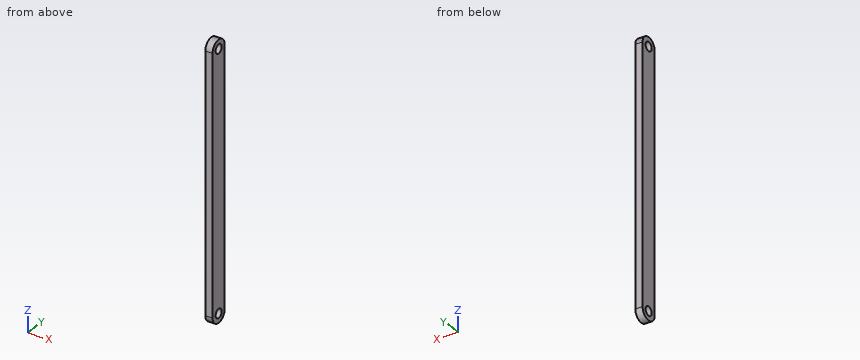
Autodesk Inventor part; units mm, degrees
ref_plane "YZ Plane" through (0, 0, 0) normal (1, 0, 0) x (0, 1, 0)
ref_plane "XZ Plane" through (0, 0, 0) normal (0, 1, 0) x (-1, 0, 0)
ref_plane "XY Plane" through (0, 0, 0) normal (0, 0, 1) x (1, 0, 0)
sketch "Sketch1" plane through (0, 0, 0) normal (1, 0, 0) x (0, 1, 0)
  line L0 (0, 0) -> (0, -70)
  arc A0 (2.5, 0) -> (-2.5, 0) centre (0, 0) ccw
  arc A1 (-2.5, -70) -> (2.5, -70) centre (0, -70) ccw
  line L1 (2.5, 0) -> (2.5, -70)
  line L2 (-2.5, 0) -> (-2.5, -70)
  circle A2 centre (0, 0) radius 1.25
  circle A3 centre (0, -70) radius 1.25
  dimension "d0" = 70
  dimension "d1" = 5
  dimension "d2" = 5
  dimension "d3" = 2.5
  dimension "d4" = 2.5
extrude "Extrusion1" add sketch "Sketch1" along normal blind 2
properties part number "base3"
Here's how the part is built. I have some questions about the finished solid (model axes, mm). Round coordinates to 2 decimals unless told otherwise and drop trailing zeros. Order: outer loops, then holes, each group sorted by start corner. A loop starts at its lowest first (then second) coordinate and runs counter-clockwise, first axis right, second up. Notation, with made-up numbers: (-6, 32) -> (31, 32) arc R30 cw to (31, 67) -> close; hole circle Ø9 at (-7.75, 20.5). An arc over 180 degrees is marked (long way). Use CSV: the item, a comma, the result in double quotes.
1. I want a section at B-B on x = 0.95. List the corners of the cut face in (y, z) for me, and give its area (3 significant figures).
Recorded:
outline,"(-2.5, -70) arc R2.5 ccw to (2.5, -70) -> (2.5, 0) arc R2.5 ccw to (-2.5, 0) -> close; hole circle Ø2.5 at (0, -70); hole circle Ø2.5 at (0, 0)"
area,"360 mm2"
2. I want a section at A-A on y = 0. List the corners of the cut face in (x, z) for me, and give its area (3 significant figures).
Recorded:
outline,"(0, -72.5) -> (2, -72.5) -> (2, -71.25) -> (0, -71.25) -> close; (0, -68.75) -> (2, -68.75) -> (2, -1.25) -> (0, -1.25) -> close; (0, 1.25) -> (2, 1.25) -> (2, 2.5) -> (0, 2.5) -> close"
area,"140 mm2"
3. I'm going to push a flat-ended pin straight in: P1, Ø2, axis at y = 0, z = 0, coming from the -X side. Where does the tip first touch, or does it pass through?
Recorded:
P1,"passes through"
4. I need wall thicknesses on line 1 along Z through (x, y) = (1.4, 0); line 2 along Y through (x, z) = (1.05, -70); line 3 along Y through (x, z) = (0.6, -0.5). Which ranges of each line are inside material? Lowest first, please.
Recorded:
line 1,"z = -72.5 to -71.25, -68.75 to -1.25, 1.25 to 2.5"
line 2,"y = -2.5 to -1.25, 1.25 to 2.5"
line 3,"y = -2.5 to -1.15, 1.15 to 2.5"
